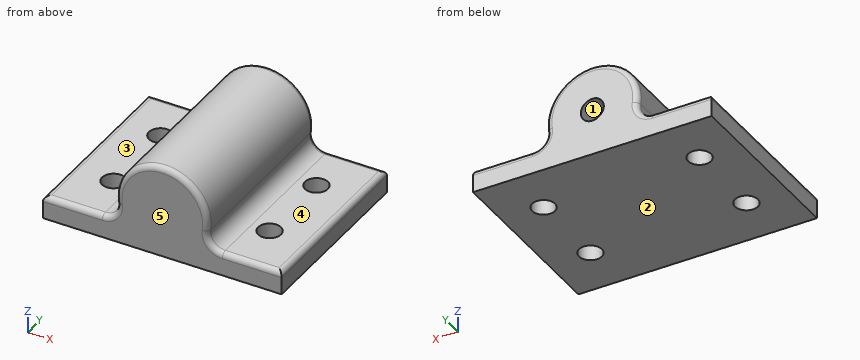
```python
from build123d import *

# Parameters (mm, degrees)
SKETCH1_R           = 6.35
BOSS_EXTRUDE1_DEPTH = 12.7
SKETCH2_W           = 33.02
SKETCH2_H           = 3.175
BOSS_EXTRUDE2_DEPTH = 25.4
CUT_EXTRUDE1_REACH  = 5.175
SKETCH4_R           = 1.5875
SKETCH5_R           = 1.5875
CUT_EXTRUDE2_DEPTH  = 19.05
FILLET2_R           = 2.032
FILLET3_R           = 0.762


with BuildPart() as part:
    # Sketch1 → Boss-Extrude1 (new body, symmetric)
    with BuildSketch(Plane(origin=(0, 0, 0), x_dir=(1, 0, 0), z_dir=(0, 1, 0))):
        Circle(SKETCH1_R)
    extrude(amount=BOSS_EXTRUDE1_DEPTH, both=True)

    # Sketch2 → Boss-Extrude2 (add)
    with BuildSketch(Plane.XZ.offset(12.7)):
        with Locations((0, -4.826)):
            Rectangle(SKETCH2_W, SKETCH2_H)
    extrude(amount=-BOSS_EXTRUDE2_DEPTH)

    # Sketch4 → Cut-Extrude1 (cut, up to next)
    with BuildSketch(Plane.XY.offset(-3.2385), mode=Mode.PRIVATE) as cut_extrude1_sk1:
        with Locations((10.795, 5.6515)):
            Circle(SKETCH4_R)
    cut_extrude1_tool1 = extrude(cut_extrude1_sk1.sketch, amount=-CUT_EXTRUDE1_REACH, mode=Mode.PRIVATE) & part.part
    add(cut_extrude1_tool1.solids().sort_by_distance((10.795, 5.6515, -3.2385))[0], mode=Mode.SUBTRACT)
    # Sketch4 → Cut-Extrude1 (cut, up to next)
    with BuildSketch(Plane.XY.offset(-3.2385), mode=Mode.PRIVATE) as cut_extrude1_sk2:
        with Locations((10.795, -5.6515)):
            Circle(SKETCH4_R)
    cut_extrude1_tool2 = extrude(cut_extrude1_sk2.sketch, amount=-CUT_EXTRUDE1_REACH, mode=Mode.PRIVATE) & part.part
    add(cut_extrude1_tool2.solids().sort_by_distance((10.795, -5.6515, -3.2385))[0], mode=Mode.SUBTRACT)
    # Sketch4 → Cut-Extrude1 (cut, up to next)
    with BuildSketch(Plane.XY.offset(-3.2385), mode=Mode.PRIVATE) as cut_extrude1_sk3:
        with Locations((-10.795, -5.6515)):
            Circle(SKETCH4_R)
    cut_extrude1_tool3 = extrude(cut_extrude1_sk3.sketch, amount=-CUT_EXTRUDE1_REACH, mode=Mode.PRIVATE) & part.part
    add(cut_extrude1_tool3.solids().sort_by_distance((-10.795, -5.6515, -3.2385))[0], mode=Mode.SUBTRACT)
    # Sketch4 → Cut-Extrude1 (cut, up to next)
    with BuildSketch(Plane.XY.offset(-3.2385), mode=Mode.PRIVATE) as cut_extrude1_sk4:
        with Locations((-10.795, 5.6515)):
            Circle(SKETCH4_R)
    cut_extrude1_tool4 = extrude(cut_extrude1_sk4.sketch, amount=-CUT_EXTRUDE1_REACH, mode=Mode.PRIVATE) & part.part
    add(cut_extrude1_tool4.solids().sort_by_distance((-10.795, 5.6515, -3.2385))[0], mode=Mode.SUBTRACT)

    # Sketch5 → Cut-Extrude2 (cut)
    with BuildSketch(Plane(origin=(0, 12.7, 0), x_dir=(1, 0, 0), z_dir=(0, 1, 0))):
        Circle(SKETCH5_R)
    extrude(amount=-CUT_EXTRUDE2_DEPTH, mode=Mode.SUBTRACT)

    # Fillet2
    fillet2_edges = [part.edges().sort_by_distance(p)[0] for p in [
        (-5.462107446, 0, -3.2385),
        (5.462107446, 0, -3.2385),
    ]]
    fillet(fillet2_edges, radius=FILLET2_R)

    # Fillet3
    fillet3_edges = [part.edges().sort_by_distance(p)[0] for p in [
        (12.402357042, -12.7, -3.2385),
        (0, 12.7, 6.35),
        (0, -12.7, 6.35),
        (-12.402357042, 12.7, -3.2385),
        (-12.402357042, -12.7, -3.2385),
        (-6.757939343, -12.7, -2.535916185),
        (-6.757939343, 12.7, -2.535916185),
        (6.757939343, 12.7, -2.535916185),
        (6.757939343, -12.7, -2.535916185),
        (-16.51, 0, -3.2385),
        (12.402357042, 12.7, -3.2385),
        (16.51, 0, -3.2385),
    ]]
    fillet(fillet3_edges, radius=FILLET3_R)


solid = part.part
```
Geometry check sheet. Reference: the model listing, model coordinates, mm. Face numbers are marked on the shaded views. A direction names the side the tool comes from. Round coordinates to 2 decimals unless told otherwise and drop trailing zeros. Loops run counter-clockwise (first coordinate to the right, second up) from the corner with the lowest first, then second, coordinate; pieces in that order, holes last. Notation, with made-up numbers: (-17, 62) - (-5, 62) arc R27 ccw to (-5, 96) - close; hole circle Ø11 at (-10.75, -33). An arc over 180 degrees is marked (long way). Use a Markdown table: item, result.
Q1. Access from +Z, -Z, +X, -X, +Y, -Y to the whole of each face (thin tool, end or side, straight path). Record for the marked faces 4 and 5.
Solutions:
| item | result |
|---|---|
| face 4 | +Z, +X, +Y, -Y |
| face 5 | +Z, -Z, +X, -X, -Y |
Q2. Cross-section at C-C on y = -11. Record the cut outline in (x, z).
Solutions:
| item | result |
|---|---|
| outline | (-16.51, -6.41) - (16.51, -6.41) - (16.51, -4) arc R0.76 ccw to (15.75, -3.24) - (8.29, -3.24) arc R2.03 cw to (6.28, -0.91) arc R6.35 ccw (long way) to (-6.28, -0.91) arc R2.03 cw to (-8.29, -3.24) - (-15.75, -3.24) arc R0.76 ccw to (-16.51, -4) - close |
Q3. Cross-section at B-B on x = -10. Record the cut outline in (y, z).
Solutions:
| item | result |
|---|---|
| outline | (-12.7, -6.41) - (-7.03, -6.41) - (-7.03, -3.24) - (-11.94, -3.24) arc R0.76 ccw to (-12.7, -4) - close; (-4.28, -6.41) - (4.28, -6.41) - (4.28, -3.24) - (-4.28, -3.24) - close; (7.03, -6.41) - (12.7, -6.41) - (12.7, -4) arc R0.76 ccw to (11.94, -3.24) - (7.03, -3.24) - close |
Q4. Draft check along Z on the marked faces 1, 2 and 3. Enter one of: released by +Z, released by -Z, zero draft, split by the parting line, or undercut.
Solutions:
| item | result |
|---|---|
| face 1 | undercut |
| face 2 | released by -Z |
| face 3 | released by +Z |
Q5. Cross-section at A-A on z = -5.25. Record the cut outline in (x, y) (1 decimal), plus the area to 3 significant figures.
Solutions:
| item | result |
|---|---|
| outline | (-16.5, -12.7) - (16.5, -12.7) - (16.5, 12.7) - (-16.5, 12.7) - close; hole circle Ø3.2 at (-10.8, -5.7); hole circle Ø3.2 at (-10.8, 5.7); hole circle Ø3.2 at (10.8, -5.7); hole circle Ø3.2 at (10.8, 5.7) |
| area | 807 mm2 |
Q6. Material ranges on line 1 (Z direction, x = -14.5, y = 1); line 2 (X direction, y = 6, z = 0); line 3 (X direction, y = 5, z = -4.25), recorded low to high.
Solutions:
| item | result |
|---|---|
| line 1 | z = -6.41 to -3.24 |
| line 2 | x = -6.35 to -1.59, 1.59 to 6.35 |
| line 3 | x = -16.51 to -12.24, -9.35 to 9.35, 12.24 to 16.51 |
Q7. Cross-section at D-D on x = 0. Record the cut outline in (y, z), plus the area to 3 significant figures.
Solutions:
| item | result |
|---|---|
| outline | (-12.7, -6.41) - (12.7, -6.41) - (12.7, -1.59) - (-6.35, -1.59) - (-6.35, 1.59) - (12.7, 1.59) - (12.7, 5.59) arc R0.76 ccw to (11.94, 6.35) - (-11.94, 6.35) arc R0.76 ccw to (-12.7, 5.59) - close |
| area | 263 mm2 |
Q8. Go/stop test with flat-tipped pins: P1, Ø2, axis at y = 9, z = -0.5, coming from the -X side; P2, Ø12, axis at x = 1, y = 8, coming from the +Z side; P3, Ø8, axis at x = 11, y = -0.5, coming from the +Z side; P4, Ø1.5, axis at y = 6, z = -1.5, coming from the +X side. Record where each tip stops, or that it passes through.
Solutions:
| item | result |
|---|---|
| P1 | stops at x = -6.35 |
| P2 | stops at z = 6.35 |
| P3 | stops at z = -2.77 |
| P4 | stops at x = 6.55 |
